from build123d import *

# Parameters (mm, degrees)
F0_W     = 320
F0_H     = 370
F1_DEPTH = 70
F2_W     = 282
F2_H     = 332
F3_DEPTH = 51
F4_W     = 342
F4_H     = 140
F4_W_2   = 320
F4_H_2   = 70
F5_DEPTH = 19
F6_W     = 100
F6_H     = 30
F7_DEPTH = 19


with BuildPart() as f1:
    # F0 (on Top) → F1 (new body)
    with BuildSketch(Plane.XY):
        Rectangle(F0_W, F0_H)
    extrude(amount=F1_DEPTH)

    # F2 (on face) → F3 (cut)
    with BuildSketch(Plane.XY.offset(70)):
        Rectangle(F2_W, F2_H)
    extrude(amount=-F3_DEPTH, mode=Mode.SUBTRACT)

    # F4 (on face) → F5 (join)
    with BuildSketch(Plane.XZ.offset(185)):
        with Locations((0, 35)):
            Rectangle(F4_W, F4_H)
        with Locations((0, 35)):
            Rectangle(F4_W_2, F4_H_2, mode=Mode.SUBTRACT)
        with Locations((0, 35)):
            Rectangle(F4_W_2, F4_H_2)
    extrude(amount=F5_DEPTH)

    # F6 (on face) → F7 (join)
    with BuildSketch(Plane.XZ.offset(204)):
        with Locations((0, 35)):
            Rectangle(F6_W, F6_H)
    extrude(amount=F7_DEPTH)


solid = f1.part
Source: CAD feature listing. Evaluate the final solid. Frame: model axes, mm. A direction names the side the tool comes from. Round coordinates to 2 decimals unless told otherwise and drop trailing zeros. Write each loop counter-clockwise with the first axis right and the second up, starting at its lowest first coordinate (ties: lowest second). Pieces come first, ordered by that corner, then holes. Notation, with made-up numbers: M -33.5,-38.75 L -9.5,-38.75 A21 ccw -9.5,-27.75 Z; hole C -14,12 d2. An arc over 180 degrees is marked long. One line per item, written item: value. Start each with the question number.
Item 1: Section query D-D (z = 55.5). Return the cut outline in (x, y), plus the area to 3 significant figures.
Item 2: Ray query, L1, parallel to X at y = 131.5, z = 68; L2, parallel to Y at x = -112.5, z = 23.5; L3, parallel to Y at x = 23, z = 22. Return the intervals inside material, ascending. Write a range as from..to.
Item 3: Mould query, pull axis X, two halves, no side actions, for faces 5 (the flat face through (-2, -194, -35)), 6 (the flat face through (-141, -2, 45)), 7 (the flat face through (50, -213, 35)), 8 (the flat face through (-160, -3, 35)). Classes: pulls with the +X half, pulls with the -X half, needs draft (parallel to the pull), parting line crosses it, or undercut.
Item 4: Section query C-C (y = 140.5). Return the cut outline in (x, z), plus the area to 3 significant figures.
Item 5: Pin query (flat end, axial travel): pin 1 (15.5 mm diameter, centred on y = -68.5, z = 39, fed in from -X); pin 2 (1 mm diameter, centred on x = -115, y = -38, fed in from -Z); pin 3 (5.5 mm diameter, centred on x = -9, y = -212.5, fed in from -Z); pin 4 (21 mm diameter, centred on y = -213, z = 40.5, fed in from +X). Return the tip coordinate at first contact, or that it passes through.
Item 6: Set-up query: faces 1 (the flat face through (-1, -213, 50)), 2 (the flat face through (160, -3, 35)), 3 (the flat face through (-1, -213, 20)), 4 (the flat face through (-50, -213, 35)). Return all of +Z, -Z, +X, -X, +Y, -Y with unobstructed straight access to the full face (end or side cutting, diameter ignored); none if empty.
Item 7: Section query A-A (z = 26.5). Return the cut outline in (x, y).
Item 8: Section query B-B (x = -62.5). Return the cut outline in (y, z).
Result set:
1. outline: M -171,-204 L 171,-204 L 171,-185 L 160,-185 L 160,185 L -160,185 L -160,-185 L -171,-185 Z; hole M -141,-166 L 141,-166 L 141,166 L -141,166 Z
1. area: 31,300 mm²
2. L1: x = -160..-141, 141..160
2. L2: y = -204..-166, 166..185
2. L3: y = -223..-166, 166..185
3. face 5: needs draft
3. face 6: undercut
3. face 7: pulls with the +X half
3. face 8: pulls with the -X half
4. outline: M -160,0 L 160,0 L 160,70 L 141,70 L 141,19 L -141,19 L -141,70 L -160,70 Z
4. area: 8,020 mm²
5. pin 1: stops at x = -160
5. pin 2: stops at z = 0
5. pin 3: stops at z = 20
5. pin 4: stops at x = 171
6. face 1: +Z, +X, -X, -Y
6. face 2: +Z, -Z, +X, +Y
6. face 3: -Z, +X, -X, -Y
6. face 4: +Z, -Z, -X, -Y
7. outline: M -171,-204 L -50,-204 L -50,-223 L 50,-223 L 50,-204 L 171,-204 L 171,-185 L 160,-185 L 160,185 L -160,185 L -160,-185 L -171,-185 Z; hole M -141,-166 L 141,-166 L 141,166 L -141,166 Z
8. outline: M -204,-35 L -185,-35 L -185,0 L 185,0 L 185,70 L 166,70 L 166,19 L -166,19 L -166,70 L -185,70 L -185,105 L -204,105 Z
